Part model, mm, in its own coordinate system. A direction names the side the tool comes from. Coordinates: 2 decimals unless noted, no trailing zeros. Loops run counter-clockwise (first coordinate to the right, second up) from the corner with the lowest first, then second, coordinate; pieces in that order, holes last. Notation, with made-up numbers: (-29.75, 2.25) - (-24.75, 2.25) arc R34 ccw to (-24.75, 34.25) - close; hole circle Ø11 at (84, 20.25). An arc over 180 degrees is marked (long way). Answer as CSV lines item,"result".
from build123d import *

# Parameters (mm, degrees)
BOSS_EXTRUDE1_DEPTH = 5
SKETCH2_R           = 1.2
CUT_EXTRUDE1_DEPTH  = 117.909745524
BOSS_EXTRUDE2_DEPTH = 12.879


with BuildPart() as part:
    # Sketch1 → Boss-Extrude1 (new body)
    with BuildSketch(Plane.XY):
        with BuildLine():
            Line((0, -39.4175), (0, 39.4175))
            ThreePointArc((0, 39.4175), (101.221, 0), (0, -39.4175))
        make_face()
    extrude(amount=BOSS_EXTRUDE1_DEPTH)

    # Sketch2 → Cut-Extrude1 (cut, through all)
    with BuildSketch(Plane.XY.offset(5)):
        with Locations((2.5, 19.70875)):
            Circle(SKETCH2_R)
        with Locations((2.5, 0)):
            Circle(SKETCH2_R)
        with Locations((2.5, -19.70875)):
            Circle(SKETCH2_R)
        with Locations((14.450382973, 47.941684776)):
            Circle(SKETCH2_R)
        with Locations((15.603067001, -48.610455862)):
            Circle(SKETCH2_R)
    extrude(amount=-CUT_EXTRUDE1_DEPTH, mode=Mode.SUBTRACT)

    # Sketch3 → Boss-Extrude2 (add)
    with BuildSketch(Plane.XY.offset(5)):
        with BuildLine():
            Line((27.955, -56.327452693), (27.955, -51.136357684))
            ThreePointArc((27.955, -51.136357684), (96.203818326, 1.353060418), (25.378179175, 50.30986847))
            Line((25.378179175, 50.30986847), (27.236614528, 56.131473172))
            ThreePointArc((27.236614528, 56.131473172), (101.219810829, 0.372318969), (27.955, -56.327452693))
        make_face()
    extrude(amount=BOSS_EXTRUDE2_DEPTH)


solid = part.part
Q1. Saw through at B-B (z = 8.25). Give the cut face in (x, y) (3 decimals).
Results:
outline,"(25.378, 50.31) arc R53.285 cw (long way) to (27.955, -51.136) - (27.955, -56.327) arc R58.285 ccw (long way) to (27.237, 56.131) - close"
Q2. Saw through at D-D (x = 73.5). Give the cut face in (y, z), then the cut area to 3 significant figures.
Results:
outline,"(-49.63, 0) - (49.63, 0) - (49.63, 17.88) - (43.65, 17.88) - (43.65, 5) - (-43.65, 5) - (-43.65, 17.88) - (-49.63, 17.88) - close"
area,"650 mm^2"
Q3. Wall check: L1, parallel to Y at x = 2.5, z = 2.35; L2, parallel to Z at x = 73.5, y = 27.5; L3, parallel to Y at x = 76.5, z = 11.5. Give the ranges that are in metal, low to high.
Results:
L1,"y = -41.98 to -20.91, -18.51 to -1.2, 1.2 to 18.51, 20.91 to 41.98"
L2,"z = 0 to 5"
L3,"y = -47.65 to -41.39, 41.39 to 47.65"
Q4. Saw through at A-A (x = 84). Give the cut face in (y, z), then the cut area to 3 significant figures.
Results:
outline,"(-41.36, 0) - (41.36, 0) - (41.36, 17.88) - (33.96, 17.88) - (33.96, 5) - (-33.96, 5) - (-33.96, 17.88) - (-41.36, 17.88) - close"
area,"604 mm^2"
Q5. Which spindle directions (+Z, -Z, +X, -X, +Y, -Y) get a long thin tool onto all of the face, cutting with end or side? Do faces 4 (the face through (27.955, -54, 11)), 5 (the face through (96.22, -0.05, 11.35)), 6 (the face through (3.645, 0.36, 2.535)). Say none if no direction does.
Results:
face 4,"+Z, -X, -Y"
face 5,"+Z"
face 6,"+Z, -Z"
Q6. Two-plate mould, pull along Y, no slides. Class faces 1 (the face through (51, 1, 0)), 2 (the face through (26.3, 53.2, 11.3)), 3 (the face through (15.45, -47.42, 2.54)): released by +Y, released by -Y, zero draft, split by the parting line, or undercut.
Results:
face 1,"zero draft"
face 2,"released by +Y"
face 3,"undercut"
Q7. Saw through at C-C (y = -4.5). Give the cut face in (x, z), then the cut area to 3 significant figures.
Results:
outline,"(0, 0) - (101.05, 0) - (101.05, 17.88) - (96.03, 17.88) - (96.03, 5) - (0, 5) - close"
area,"570 mm^2"
Q8. Flat gauge pins, fed straight in: pin 1 (1.5 mm diameter, centred on x = 13, y = -19.5, fed in from -Z); pin 2 (5 mm diameter, centred on y = 23.5, z = 14.5, fed in from -X); pin 3 (1 mm diameter, centred on y = -12, z = 12, fed in from -X); pin 4 (4 mm diameter, centred on y = -27.5, z = 10.5, fed in from -X). Where does each tip first touch, or does it go through?
Results:
pin 1,"stops at z = 0"
pin 2,"stops at x = 89.45"
pin 3,"stops at x = 94.73"
pin 4,"stops at x = 87.31"
